```python
from build123d import *

# Parameters (mm, degrees)
AUFSATZ_LINEAR_AUSTRAGEN1_DEPTH = 8.5
CUT_EXTRUDE4_DEPTH              = 5
SKETCH2_R                       = 1.5
CUT_EXTRUDE5_DEPTH              = 9.5
CUT_EXTRUDE6_DEPTH              = 9.5
SKETCH3_W                       = 3.6
SKETCH3_H                       = 7.3
CUT_EXTRUDE9_DEPTH              = 7.95
SKETCH4_R                       = 2.25
CUT_EXTRUDE10_DEPTH             = 20
BOSS_EXTRUDE1_START             = -20
BOSS_EXTRUDE1_DEPTH             = 10
AUFSATZ_LINEAR_AUSTRAGEN2_DEPTH = 3.6
SCHNITT_LINEAR_AUSTRAGEN1_DEPTH = 3.6
LPATTERN1_COUNT                 = 3
LPATTERN1_PITCH                 = 35
SKIZZE4_R                       = 3.25
SCHNITT_LINEAR_AUSTRAGEN2_DEPTH = 2


with BuildPart() as part:
    # Skizze1 → Aufsatz-Linear austragen1 (new body)
    with BuildSketch(Plane.XY):
        with BuildLine():
            Line((120.133333333, 7.998888812), (0.166666667, 9.998611015))
            ThreePointArc((0.166666667, 9.998611015), (-10, 0), (0.166666667, -9.998611015))
            Line((0.166666667, -9.998611015), (120.133333333, -7.998888812))
            Line((120.133333333, -7.998888812), (120.133333333, 7.998888812))
        make_face()
    extrude(amount=AUFSATZ_LINEAR_AUSTRAGEN1_DEPTH)

    # Sketch1 → Cut-Extrude4 (cut)
    with BuildSketch(Plane.XY.offset(8.5)):
        with BuildLine():
            Line((-4.200128323, -6.276826928), (4.200128323, -6.276826928))
            ThreePointArc((4.200128323, -6.276826928), (4.808454435, -4.808197778), (6.277083585, -4.199871666))
            Line((6.277083585, -4.199871666), (7.877083585, -4.199871666))
            Line((7.877083585, -4.199871666), (17.44738825, -2.459668071))
            ThreePointArc((17.44738825, -2.459668071), (19.500137785, 0), (17.44738825, 2.459668071))
            Line((17.44738825, 2.459668071), (7.877083585, 4.199871666))
            Line((7.877083585, 4.199871666), (6.277083585, 4.199871666))
            ThreePointArc((6.277083585, 4.199871666), (4.808454435, 4.808197778), (4.200128323, 6.276826928))
            Line((4.200128323, 6.276826928), (-4.200128323, 6.276826928))
            ThreePointArc((-4.200128323, 6.276826928), (-4.808454435, 4.808197778), (-6.277083585, 4.199871666))
            Line((-6.277083585, 4.199871666), (-6.277083585, -4.199871666))
            ThreePointArc((-6.277083585, -4.199871666), (-4.808454435, -4.808197778), (-4.200128323, -6.276826928))
        make_face()
    extrude(amount=-CUT_EXTRUDE4_DEPTH, mode=Mode.SUBTRACT)

    # Sketch2 → Cut-Extrude5 (cut, through all)
    with BuildSketch(Plane(origin=(0, 0, 0), x_dir=(-1, 0, 0), z_dir=(0, 0, -1))):
        Circle(SKETCH2_R)
    extrude(amount=-CUT_EXTRUDE5_DEPTH, mode=Mode.SUBTRACT)

    # Skizze2 → Cut-Extrude6 (cut, through all)
    with BuildSketch(Plane.XY.offset(8.5)):
        with BuildLine():
            Line((90.183296296, 2.997361391), (30.066666667, 3.999444406))
            ThreePointArc((30.066666667, 3.999444406), (26, 0), (30.066666667, -3.999444406))
            Line((30.066666667, -3.999444406), (90.183296296, -2.997361391))
            ThreePointArc((90.183296296, -2.997361391), (93.131111111, 0), (90.183296296, 2.997361391))
        make_face()
    extrude(amount=-CUT_EXTRUDE6_DEPTH, mode=Mode.SUBTRACT)

    # Sketch3 → Cut-Extrude9 (cut)
    with BuildSketch(Plane.XY.offset(8.5)):
        with Locations((108.333333333, 0)):
            Rectangle(SKETCH3_W, SKETCH3_H)
    extrude(amount=-CUT_EXTRUDE9_DEPTH, mode=Mode.SUBTRACT)

    # Sketch4 → Cut-Extrude10 (cut)
    with BuildSketch(Plane(origin=(120.133333333, 0, 0), x_dir=(0, 0, -1), z_dir=(1, 0, 0))):
        with Locations((-4.25, 0)):
            Circle(SKETCH4_R)
    extrude(amount=-CUT_EXTRUDE10_DEPTH, mode=Mode.SUBTRACT)

    # Sketch5 → Boss-Extrude1 (add)
    with BuildSketch(Plane(origin=(119.966666667, -1.999722203, 0), x_dir=(0, 0, -1), z_dir=(0.999861101, -0.016666667, 0)).offset(BOSS_EXTRUDE1_START)):
        Polygon((0, 10), (0, 13), (-1, 14), (-8, 14), (-8, 13), (-4.541308146, 11), (-4.541308146, 13.041308146), (-3.041308146, 13.041308146), (-1.5, 11.5), (-1.5, 10), align=None)
    boss_extrude1 = extrude(amount=-BOSS_EXTRUDE1_DEPTH)

    # Skizze3 → Aufsatz-Linear austragen2 (add)
    with BuildSketch(Plane(origin=(106.533333333, 0, 0), x_dir=(0, 0, -1), z_dir=(1, 0, 0))):
        Polygon((-0.55, 3.65), (-3.171985448, 3.65), (-0.55, 2.136195996), align=None)
        Polygon((-0.55, -3.65), (-0.55, -2.136195996), (-3.171985448, -3.65), align=None)
    extrude(amount=AUFSATZ_LINEAR_AUSTRAGEN2_DEPTH)

    # Skizze3_3 → Schnitt-Linear austragen1 (cut)
    with BuildSketch(Plane(origin=(106.533333333, 0, 0), x_dir=(0, 0, -1), z_dir=(1, 0, 0))):
        Polygon((-5.328014552, 3.65), (-4.25, 4.272391992), (-8.5, 4.272391992), (-8.5, 3.65), align=None)
        Polygon((-3.171985448, 3.65), (-4.25, 4.272391992), (-5.328014552, 3.65), align=None)
        Polygon((-3.171985448, -3.65), (-5.328014552, -3.65), (-4.25, -4.272391992), align=None)
        Polygon((-5.328014552, -3.65), (-8.5, -3.65), (-8.5, -4.272391992), (-4.25, -4.272391992), align=None)
    extrude(amount=SCHNITT_LINEAR_AUSTRAGEN1_DEPTH, mode=Mode.SUBTRACT)

    # LPattern1: Boss-Extrude1 ×3
    with Locations(*[Vector(-0.999861101, 0.016666667, 0) * (i * LPATTERN1_PITCH) for i in range(1, LPATTERN1_COUNT)]):
        add(boss_extrude1)

    # Skizze4 → Schnitt-Linear austragen2 (cut)
    with BuildSketch(Plane(origin=(0, 0, 0), x_dir=(-1, 0, 0), z_dir=(0, 0, -1))):
        Circle(SKIZZE4_R)
    extrude(amount=-SCHNITT_LINEAR_AUSTRAGEN2_DEPTH, mode=Mode.SUBTRACT)


solid = part.part
```
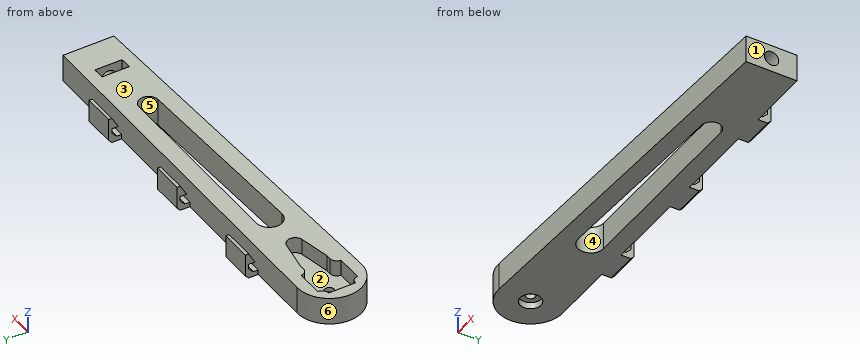
The model under review builds one solid part; all positions refer to its coordinate system, in mm. Face numbers are marked on the shaded views. A direction names the side the tool comes from. Give positions to 0.01 mm unless a question says otherwise; leave off trailing zeros. Write each loop counter-clockwise with the first axis right and the second up, starting at its lowest first coordinate (ties: lowest second). Pieces come first, ordered by that corner, then holes.
(1) The part is to be moulded in two halves that separate along Y. For the marked faces 3, 4, 5 and 6, say which applies: released by +Y, released by -Y, zero draft, split by the parting line, or undercut.
(2) Consider section B-B, the plane x = 57.5. Give the boundary of the cut face in (y, z).
(3) Consider section D-D, the plane x = 15. Give the boundary of the cut face in (y, z), and give its area (3 significant figures).
(4) Tool access review of the marked faces 1 and 2: name each direction out of +Z, -Z, +X, -X, +Y, -Y from which nothing blocks a thin tool from reaching the whole face with its end or side.
(5) For P1, Ø0.6, axis at x = 61, y = 12.5, coming from the +Z side; P2, Ø4, axis at y = 8, z = 3.5, coming from the -X side; P3, Ø2.5, axis at x = 0, y = 0, coming from the -Z side; P4, Ø5, axis at x = -1.5, y = 0, coming from the -Z side, all flat-tipped, find the tip position at first contact; note any pin that passes through.
(6) Consider section C-C, the plane x = 34. Give the boundary of the cut face in (y, z), and give its area (3 significant figures).
(7) To check wall thickness, follow L1, parallel to X at y = 11.75, z = 1; L2, parallel to X at y = 1.5, z = 7; L3, parallel to Y at x = 0, z = 2.7. State the ranges of each line that lie inside material, in increasing order.
(8) Consider section A-A, the plane y = 0. Give the number of separate pieces and of enclosed holes in the cut face, and give its area (3 significant figures).
Returned:
1. face 3: zero draft
1. face 4: undercut
1. face 5: undercut
1. face 6: split by the parting line
2. outline: (-9.04, 0) - (-3.54, 0) - (-3.54, 8.5) - (-9.04, 8.5) - close; (3.54, 0) - (12.04, 0) - (13.04, 1) - (13.04, 8) - (12.04, 8) - (10.04, 4.54) - (12.08, 4.54) - (12.08, 3.04) - (10.54, 1.5) - (9.04, 1.5) - (9.04, 8.5) - (3.54, 8.5) - close
3. outline: (-9.75, 0) - (9.75, 0) - (9.75, 8.5) - (2.9, 8.5) - (2.9, 3.5) - (-2.9, 3.5) - (-2.9, 8.5) - (-9.75, 8.5) - close
3. area: 137 mm2
4. face 1: +Z, -Z, +X, +Y, -Y
4. face 2: +Z
5. P1: stops at z = 8
5. P2: stops at x = -8
5. P3: passes through
5. P4: stops at z = 0
6. outline: (-9.43, 0) - (-3.93, 0) - (-3.93, 8.5) - (-9.43, 8.5) - close; (3.93, 0) - (9.43, 0) - (9.43, 8.5) - (3.93, 8.5) - close
6. area: 93.5 mm2
7. L1: x = 20.18 to 30.18, 55.19 to 65.19, 90.19 to 100.19
7. L2: x = -9.89 to -6.28, 19 to 26.29, 92.73 to 106.53, 110.13 to 120.13
7. L3: y = -10 to -1.5, 1.5 to 10
8. separate pieces: 4
8. enclosed holes: 0
8. area: 287 mm2
